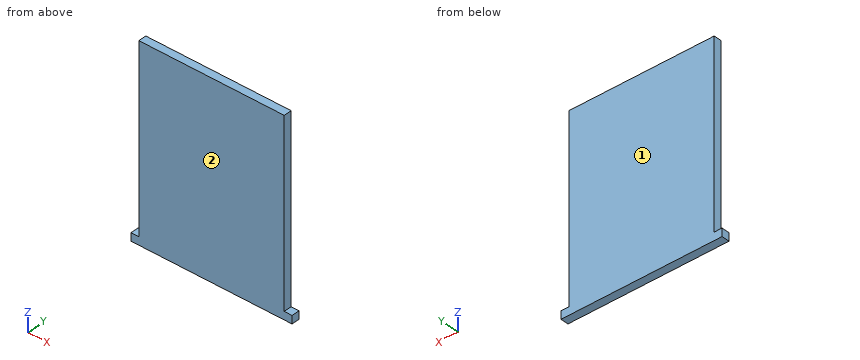
Autodesk Inventor part; units mm, degrees
ref_plane "YZ Plane" through (0, 0, 0) normal (1, 0, 0) x (0, 1, 0)
ref_plane "XZ Plane" through (0, 0, 0) normal (0, 1, 0) x (-1, 0, 0)
ref_plane "XY Plane" through (0, 0, 0) normal (0, 0, 1) x (1, 0, 0)
sketch "Sketch1" plane through (0, 0, 0) normal (0, 1, 0) x (-1, 0, 0)
  line L0 (0, 0) -> (6, 0)
  line L1 (6, 0) -> (6, -6)
  line L2 (6, -6) -> (0, -6)
  line L3 (0, -6) -> (0, 0)
  line L4 (0, -6) -> (-55, -6)
  line L5 (-55, -6) -> (-55, 138)
  line L6 (-55, 138) -> (0, 138)
  line L7 (0, 138) -> (0, -6)
  dimension "d0" = 6
  dimension "d1" = 6
  dimension "d2" = 55
  dimension "d3" = 144
extrude "Extrusion1" add sketch "Sketch1" along normal blind 6
mirror "Mirror1" about plane through (55, 0, 138) normal (1, 0, 0) of "Extrusion1"
properties part number "wall 4 for sorting"
Verification items for the finished model (mm, model axes). Face numbers are marked on the shaded views. Give positions to 0.01 mm unless a question says otherwise; leave off trailing zeros. Loops run counter-clockwise (first coordinate to the right, second up) from the corner with the lowest first, then second, coordinate; pieces in that order, holes last.
1. Material ranges on probe 1 along X at (y, z) = (0.95, 123.5), recorded low to high.
Derived:
probe 1: x = 0 to 110
2. Cross-section at A-A on y = 1.75. Record the cut outline in (x, z).
Derived:
outline: (-6, -6) - (116, -6) - (116, 0) - (110, 0) - (110, 138) - (0, 138) - (0, 0) - (-6, 0) - close
3. Release check for a two-part mould opening along Y. For the marked faces 1 and 2 record: +Y half, -Y half, draft (parallel to the pull), parting line (faces both ways), or undercut.
Derived:
face 1: +Y half
face 2: -Y half
4. Go/stop test with flat-tipped pins: P1, Ø1.8, axis at x = 112, y = 2.5, coming from the +Z side; P2, Ø3, axis at y = 2.5, z = 40.5, coming from the +X side. Record where each tip stops, or that it passes through.
Derived:
P1: stops at z = 0
P2: stops at x = 110
5. Cross-section at B-B on z = 15.5. Record the cut outline in (x, y).
Derived:
outline: (0, 0) - (110, 0) - (110, 6) - (0, 6) - close
